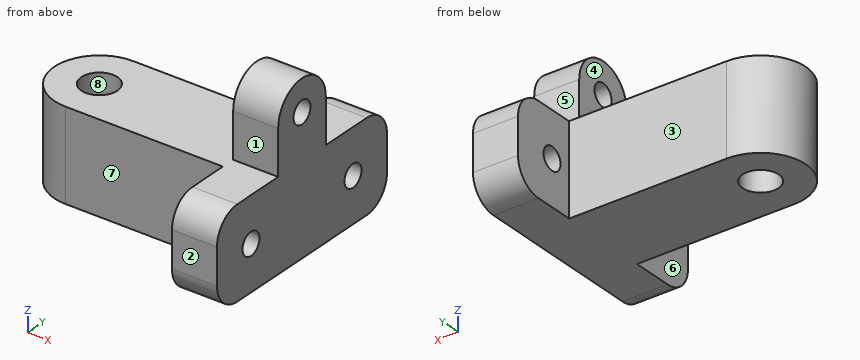
Autodesk Inventor part; units mm, degrees
ref_plane "YZ Plane" through (0, 0, 0) normal (1, 0, 0) x (0, 1, 0)
ref_plane "XZ Plane" through (0, 0, 0) normal (0, 1, 0) x (-1, 0, 0)
ref_plane "XY Plane" through (0, 0, 0) normal (0, 0, 1) x (1, 0, 0)
sketch "Sketch1" plane through (0, 0, 0) normal (0, 0, 1) x (1, 0, 0)
  line L0 (0, 0) -> (-35, 0) construction
  circle A0 centre (-35, 0) radius 4
  line L1 (10, 25) -> (0, 25)
  line L2 (0, 25) -> (0, -25)
  line L3 (0, -25) -> (10, -25)
  line L4 (10, -25) -> (10, 25)
  line L5 (0, 0) -> (-35, 0) construction
  line L6 (0, 10) -> (-35, 10)
  line L7 (-35, -10) -> (0, -10)
  arc A1 (0, -10) -> (0, 10) centre (0, 0) ccw
  arc A2 (-35, 10) -> (-35, -10) centre (-35, 0) ccw
  point P0 (-17.5, 0)
  dimension "d0" = 8
  dimension "d1" = 35
  dimension "d2" = 50
  dimension "d3" = 10
  dimension "d4" = 10
extrude "Extrusion1" add sketch "Sketch1" along normal blind 20
sketch "Sketch2" plane through (10, -25, 0) normal (1, 0, 0) x (0, 0, -1)
  line L0 (0, 50) -> (-20, 50) construction
  line L1 (-10, 50) -> (-10, 40) construction
  line L2 (0, 0) -> (-20, 0) construction
  line L3 (-10, 0) -> (-10, 10) construction
  circle A0 centre (-10, 40) radius 2.5
  circle A1 centre (-10, 10) radius 2.5
  point P0 (0, 25)
  dimension "d7" = 5
  dimension "d8" = 10
extrude "Extrusion2" cut sketch "Sketch2" against normal through all
fillet "Fillet1" radius 6 4 edges at (5, 25, 20) (5, 25, 0) (5, -25, 20) (5, -25, 0)
sketch "Sketch3" plane through (10, -19, 0) normal (1, 0, 0) x (0, 0, -1)
  line L0 (-20, 15) -> (-20, 23)
  line L1 (-20, 19) -> (-30, 19) construction
  line L2 (-20, 26) -> (-30, 26)
  line L3 (-30, 12) -> (-20, 12)
  arc A0 (-20, 12) -> (-20, 26) centre (-20, 19) ccw
  arc A1 (-30, 26) -> (-30, 12) centre (-30, 19) ccw
  circle A2 centre (-30, 19) radius 2.5
  point P0 (0, 19)
  point P1 (-25, 19)
  dimension "d12" = 5
  dimension "d13" = 7
  dimension "d14" = 10
extrude "Extrusion3" add sketch "Sketch3" against normal blind 10
properties part number "frame mount 2"
Part model, mm, in its own coordinate system. Face numbers are marked on the shaded views. A direction names the side the tool comes from. Coordinates: 2 decimals unless noted, no trailing zeros. Order: outer loops, then holes, each group sorted by start corner. A loop starts at its lowest first (then second) coordinate and runs counter-clockwise, first axis right, second up. Notation, with made-up numbers: M 74.5,57 L 79.5,57 A25 cw 79.5,88 Z; hole C -30,48 d4. An arc over 180 degrees is marked long. Use a Markdown table: item, result.
(1) Flat gauge pins, fed straight in: pin 1 (12 mm diameter, centred on x = 1.5, z = 20.5, fed in from +Y); pin 2 (10 mm diameter, centred on x = -11, z = 14.5, fed in from -Y); pin 3 (12 mm diameter, centred on y = -18.5, z = 14.5, fed in from -X). Where does each tip first touch, or does it go through?
A:
| item | result |
|---|---|
| pin 1 | stops at y = 24.98 |
| pin 2 | stops at y = -10 |
| pin 3 | stops at x = 0 |
(2) Probe L1, parallel to Y at x = 5.5, z = 10; L2, parallel to Y at x = 6.75, z = 30; L3, parallel to Y at x = -35, z = 8. List the from-to ranges inside material, lowest first.
A:
| item | result |
|---|---|
| L1 | y = -25 to -17.5, -12.5 to 12.5, 17.5 to 25 |
| L2 | y = -7 to -2.5, 2.5 to 7 |
| L3 | y = -10 to -4, 4 to 10 |
(3) Cut at B-B on y = 0. Write the cut outline in (x, z).
A:
| item | result |
|---|---|
| outline | M -45,0 L -39,0 L -39,20 L -45,20 Z; M -31,0 L 10,0 L 10,27.5 L 0,27.5 L 0,20 L -31,20 Z; M 0,32.5 L 10,32.5 L 10,37 L 0,37 Z |
(4) Tool access for the marked faces 1, 2, 3, 4 and 5: list every direction of +Z, -Z, +X, -X, +Y, -Y with a clear straight run to the whole face (end or side of a thin tool).
A:
| item | result |
|---|---|
| face 1 | +Z, +X, -X, -Y |
| face 2 | +Z, -Z, +X, -X, -Y |
| face 3 | +Z, -Z, -X, +Y |
| face 4 | +Z, -X, +Y, -Y |
| face 5 | +Z, +X, -X, +Y |
(5) Cut at D-D on y = 15. Write the cut outline in (x, z).
A:
| item | result |
|---|---|
| outline | M 0,0 L 10,0 L 10,7.5 L 0,7.5 Z; M 0,12.5 L 10,12.5 L 10,20 L 0,20 Z |
(6) Pull direction X, two halves, no side cores. Call the marked faces 6, 7 and 8: released by +X, released by -X, zero draft, split by the parting line, or undercut.
A:
| item | result |
|---|---|
| face 6 | released by -X |
| face 7 | zero draft |
| face 8 | undercut |
(7) Cut at C-C on x = 3.5. Write the cut outline in (y, z), then the cut area to 3 significant figures.
A:
| item | result |
|---|---|
| outline | M -25,6 A6 ccw -19,0 L 19,0 A6 ccw 25,6 L 25,14 A6 ccw 19,20 L 7,20 L 7,30 A7 ccw -7,30 L -7,20 L -19,20 A6 ccw -25,14 Z; hole C -15,10 d5; hole C 0,30 d5; hole C 15,10 d5 |
| area | 1,130 mm^2 |
(8) Cut at A-A on z = 10. Write the cut outline in (x, y).
A:
| item | result |
|---|---|
| outline | M -35,-10 L 0,-10 L 0,-12.5 L 10,-12.5 L 10,12.5 L 0,12.5 L 0,10 L -35,10 A10 ccw Z; M 0,-25 L 10,-25 L 10,-17.5 L 0,-17.5 Z; M 0,17.5 L 10,17.5 L 10,25 L 0,25 Z; hole C -35,0 d8 |
